from build123d import *

# Parameters (mm, degrees)
SKETCH_2_R        = 0.25
EXTRUDE_1_DEPTH   = 20
OTHER_START       = -19.9
OTHER_1_OUTLINE_R = 0.25
OTHER_1_DEPTH     = 8


# Read off the part's stored shape, not the designer's step: 连接点1
with BuildPart() as part:
    # 草图1 → 旋转1 (revolve)
    with BuildSketch(Plane.XY):
        with BuildLine():
            Line((3.5, 0.1), (3.5, 0))
            Line((3.5, 0), (4, 0))
            Line((4, 0), (4, 0.349678286))
            ThreePointArc((4, 0.349678286), (3.798136614, 0.837019609), (4, 1.324360933))
            Line((4, 1.324360933), (4, 15.6))
            Line((4, 15.6), (3.5, 15.6))
            Line((3.5, 15.6), (3.5, 15.5))
            Line((3.5, 15.5), (0, 15.5))
            Line((0, 15.5), (0, 0.1))
            Line((0, 0.1), (3.5, 0.1))
        make_face()
    revolve(axis=Axis((0, 0, 0), (0, 1, 0)))

    # 草图2 → 凸台-拉伸1 (add)
    with BuildSketch(Plane.XZ.offset(-0.1)):
        with Locations((-1.5, 0.094730426)):
            Circle(SKETCH_2_R)
        with Locations((1.5, 0.094730426)):
            Circle(SKETCH_2_R)
    extrude(amount=EXTRUDE_1_DEPTH)

    # 连接点1 outline → 连接点1 (cut)
    with BuildSketch(Plane(origin=(0, 0, 0), x_dir=(1, 0, 0), z_dir=(0, 1, 0)).offset(OTHER_START)):
        with Locations((1.5, -0.094730426)):
            Circle(OTHER_1_OUTLINE_R)
    extrude(amount=OTHER_1_DEPTH, mode=Mode.SUBTRACT)


solid = part.part
Source: CAD feature listing. Evaluate the final solid. Frame: model axes, mm. A direction names the side the tool comes from. Coordinates: 2 decimals unless noted, no trailing zeros. Loops run counter-clockwise (first coordinate to the right, second up) from the corner with the lowest first, then second, coordinate; pieces in that order, holes last. Notation, with made-up numbers: M 28.25,19 L 79.25,19 A24 cw 79.25,43 Z; hole C 84,73.5 d2. An arc over 180 degrees is marked long. Answer in a Markdown table with one row per item.
Q1. Draft query along X for faces 1 (the cylindrical face through (-0.867, 0.177, 3.905)), 2 (the flat face through (0, 15.5, 0)). Return one class per face: pulls with the +X half, pulls with the -X half, needs draft (parallel to the pull), parting line crosses it, or undercut.
Answers below:
| item | result |
|---|---|
| face 1 | parting line crosses it |
| face 2 | undercut |
Q2. Ray query, probe 1 along Z at (x, y) = (0, 0.05); probe 2 along Y at (x, z) = (1.75, -2); probe 3 along Y at (x, z) = (-1.25, 3.5). Return the intervals inside material, ascending. Write a range as from..to.
Answers below:
| item | result |
|---|---|
| probe 1 | z = -4..-3.5, 3.5..4 |
| probe 2 | y = 0.1..15.5 |
| probe 3 | y = 0..15.6 |
Q3. Section C-C on y = -2.5. Return the cut outline in (x, z), plus the area to 3 significant figures.
Answers below:
| item | result |
|---|---|
| outline | C -1.5,0.09 d0.5; C 1.5,0.09 d0.5 |
| area | 0.393 mm^2 |
Q4. Section D-D on y = -14. Return the cut outline in (x, z), plus the area to 3 significant figures.
Answers below:
| item | result |
|---|---|
| outline | C -1.5,0.09 d0.5 |
| area | 0.196 mm^2 |
Q5. Set-up query: faces 3 (the cylindrical face through (-0.867, 8.562, 3.905)), 4 (the flat face through (0, 0.1, 0)). Return all of +Z, -Z, +X, -X, +Y, -Y with unobstructed straight access to the full face (end or side cutting, diameter ignored); none if empty.
Answers below:
| item | result |
|---|---|
| face 3 | +Y, -Y |
| face 4 | -Y |
Q6. Section B-B on y = 4. Return the cut outline in (x, z), plus the area to 3 significant figures.
Answers below:
| item | result |
|---|---|
| outline | C 0,0 d8 |
| area | 50.3 mm^2 |
Q7. First-contact query: pin 1 (1 mm diameter, centred on y = 0, z = -1, fed in from +X); pin 2 (2 mm diameter, centred on x = 0, z = -0.5, fed in from +Y); pin 3 (2.5 mm diameter, centred on x = 0, z = -0.5, fed in from -Y). Flat tips, straight axial feed; report the tip coordinate or a pass-through.
Answers below:
| item | result |
|---|---|
| pin 1 | stops at x = 3.97 |
| pin 2 | stops at y = 15.5 |
| pin 3 | stops at y = 0.1 |
Q8. Section A-A on x = 0. Return the cut outline in (y, z).
Answers below:
| item | result |
|---|---|
| outline | M 0,-4 L 0.35,-4 A0.69 cw 1.32,-4 L 15.6,-4 L 15.6,-3.5 L 15.5,-3.5 L 15.5,3.5 L 15.6,3.5 L 15.6,4 L 1.32,4 A0.69 cw 0.35,4 L 0,4 L 0,3.5 L 0.1,3.5 L 0.1,-3.5 L 0,-3.5 Z |
